Work out the finished part from the listing and answer in its coordinate system (mm). A direction names the side the tool comes from. Coordinates: 2 decimals unless noted, no trailing zeros. Order: outer loops, then holes, each group sorted by start corner. A loop starts at its lowest first (then second) coordinate and runs counter-clockwise, first axis right, second up. Notation, with made-up numbers: (5, -22) -> (9, -22) arc R21 cw to (9, -6) -> close; hole circle Ø2 at (17.25, -20). An arc over 180 degrees is marked (long way). Use one line per item in the form item = value.
from build123d import *

# Parameters (mm, degrees)
BOSS_EXTRUDE1_DEPTH  = 15
CUT_EXTRUDE2_REACH   = 8.6
SKETCH3_R            = 1.595559434
CUT_EXTRUDE5_START   = -3.6
SKETCH3_6_R          = 1.595559434
CUT_EXTRUDE5_DEPTH   = 2.6
CUT_EXTRUDE3_REACH   = 5
SKETCH4_R            = 1.5
BOSS_EXTRUDE10_DEPTH = 2.5
CUT_EXTRUDE1_DEPTH   = 10.6


with BuildPart() as part:
    # Sketch1 → Boss-Extrude1 (new body)
    with BuildSketch(Plane.ZY.offset(20.222709888)):
        with BuildLine():
            Line((144.27017666, 37.109962519), (144.27017666, 13.209962519))
            Line((144.27017666, 13.209962519), (137.68267666, 13.209962519))
            Line((137.68267666, 13.209962519), (137.68267666, 10.209962519))
            Line((137.68267666, 10.209962519), (145.433552955, 10.209962519))
            ThreePointArc((145.433552955, 10.209962519), (146.341426982, 10.902339978), (147.27017666, 11.566452794))
            Line((147.27017666, 11.566452794), (147.27017666, 43.709962519))
            Line((147.27017666, 43.709962519), (137.67017666, 43.709962519))
            Line((137.67017666, 43.709962519), (137.67017666, 37.109962519))
            Line((137.67017666, 37.109962519), (144.27017666, 37.109962519))
        make_face()
    extrude(amount=-BOSS_EXTRUDE1_DEPTH)

    # Sketch3 → Cut-Extrude2 (cut, up to next)
    with BuildSketch(Plane.XZ.offset(-37.109962519), mode=Mode.PRIVATE) as cut_extrude2_sk1:
        with Locations((-16.635209888, 140.97017666)):
            Circle(SKETCH3_R)
    cut_extrude2_tool1 = extrude(cut_extrude2_sk1.sketch, amount=-CUT_EXTRUDE2_REACH, mode=Mode.PRIVATE) & part.part
    add(cut_extrude2_tool1.solids().sort_by_distance((-16.63521, 37.109963, 140.970177))[0], mode=Mode.SUBTRACT)

    # Sketch3<6> → Cut-Extrude5 (cut)
    with BuildSketch(Plane.XZ.offset(-37.109962519).offset(CUT_EXTRUDE5_START)):
        Polygon((-19.485209888, 139.324728393), (-16.635209888, 137.679280126), (-13.785209888, 139.324728393), (-13.785209888, 142.615624927), (-16.635209888, 144.261073195), (-19.485209888, 142.615624927), align=None)
        with Locations((-16.635209888, 140.97017666)):
            Circle(SKETCH3_6_R, mode=Mode.SUBTRACT)
        Polygon((-13.785209888, 139.324728393), (-16.635209888, 137.679280126), (-19.485209888, 139.324728393), (-19.485209888, 137.67017666), (-13.785209888, 137.67017666), align=None)
        with Locations((-16.635209888, 140.97017666)):
            Circle(SKETCH3_6_R)
    extrude(amount=CUT_EXTRUDE5_DEPTH, mode=Mode.SUBTRACT)

    # Sketch4 → Cut-Extrude3 (cut, up to next)
    with BuildSketch(Plane(origin=(0, 13.209962519, 0), x_dir=(1, 0, 0), z_dir=(0, 1, 0)), mode=Mode.PRIVATE) as cut_extrude3_sk1:
        with Locations((-16.431813353, -141.42017666)):
            Circle(SKETCH4_R)
    cut_extrude3_tool1 = extrude(cut_extrude3_sk1.sketch, amount=-CUT_EXTRUDE3_REACH, mode=Mode.PRIVATE) & part.part
    add(cut_extrude3_tool1.solids().sort_by_distance((-16.431813, 13.209963, 141.420177))[0], mode=Mode.SUBTRACT)
    # Sketch4 → Cut-Extrude3 (cut, up to next)
    with BuildSketch(Plane(origin=(0, 13.209962519, 0), x_dir=(1, 0, 0), z_dir=(0, 1, 0)), mode=Mode.PRIVATE) as cut_extrude3_sk2:
        with Locations((-9.013606422, -141.42017666)):
            Circle(SKETCH4_R)
    cut_extrude3_tool2 = extrude(cut_extrude3_sk2.sketch, amount=-CUT_EXTRUDE3_REACH, mode=Mode.PRIVATE) & part.part
    add(cut_extrude3_tool2.solids().sort_by_distance((-9.013606, 13.209963, 141.420177))[0], mode=Mode.SUBTRACT)

    # Sketch11 → Boss-Extrude10 (add)
    with BuildSketch(Plane(origin=(0, 13.209962519, 0), x_dir=(1, 0, 0), z_dir=(0, 1, 0))):
        Polygon((-18.077261621, -144.27017666), (-19.722709888, -141.42017666), (-18.077261621, -138.57017666), (-14.786365086, -138.57017666), (-13.140916819, -141.42017666), (-14.786365086, -144.27017666), (-10.659054689, -144.27017666), (-12.304502957, -141.42017666), (-10.659054689, -138.57017666), (-7.368158155, -138.57017666), (-5.722709888, -141.42017666), (-7.368158155, -144.27017666), (-5.222709888, -144.27017666), (-5.222709888, -137.68267666), (-20.222709888, -137.68267666), (-20.222709888, -144.27017666), align=None)
    extrude(amount=BOSS_EXTRUDE10_DEPTH)

    # Sketch2 → Cut-Extrude1 (cut, through all)
    with BuildSketch(Plane.XY.offset(147.27017666)):
        Polygon((-12.972709888, 43.709962519), (-5.222709888, 15.709962519), (-5.222709888, 43.709962519), align=None)
    extrude(amount=-CUT_EXTRUDE1_DEPTH, mode=Mode.SUBTRACT)


solid = part.part
(1) Straight lines are drawn through the part: line 1 along X through (y, z) = (13.5, 142.5); line 2 along Y through (x, z) = (-6.75, 143.75); line 3 along Y through (x, z) = (-9, 143.25). For each, find the intervals that lie inside material, in ascending order.
Data:
line_1 = -20.22 to -19.1, -13.76 to -11.68, -6.35 to -5.22
line_2 = 10.21 to 15.71
line_3 = 10.21 to 13.21
(2) Which of the six approach directions +Z, -Z, +X, -X, +Y, -Y give full straight-line access (tool end or side, diameter ignored) to faces 1 (the flat face through (-18.912, 14.442, 140.015)), 2 (the cylindrical face through (-9.209, 11.731, 139.933)), 3 (the flat face through (-19.485, 39, 140)), 4 (the cylindrical face through (-16.843, 37.603, 142.552))?
Data:
face_1 = none
face_2 = +Y, -Y
face_3 = -Z
face_4 = +Y
(3) Each of these flat-tipped pins is pushed along its axis until it touches: P1, Ø1.3, axis at y = 39, z = 139, coming from the +X side; P2, Ø2, axis at x = -10, y = 34.5, coming from the +Z side; P3, Ø2.5, axis at x = -9.01, z = 141.42, coming from the -Y side; P4, Ø2, axis at y = 39, z = 142, coming from the +X side. Where does it stop, or does it pass through?
Data:
P1 = -11.49
P2 = 147.27
P3 = through
P4 = -11.39
(4) Section C-C on x = -9 is taken. Write down the section's boundary in (y, z), plus the area to 4 significant figures.
Data:
outline = (10.21, 137.68) -> (15.71, 137.68) -> (15.71, 138.57) -> (13.21, 138.57) -> (13.21, 139.92) -> (10.21, 139.92) -> close; (10.21, 142.92) -> (13.21, 142.92) -> (13.21, 144.27) -> (29.36, 144.27) -> (29.36, 147.27) -> (11.57, 147.27) arc R37.1 cw to (10.21, 145.43) -> close
area = 69.15 mm²
(5) Section D-D on x = -15.5 is taken. Write down the section's boundary in (y, z).
Data:
outline = (10.21, 137.68) -> (15.71, 137.68) -> (15.71, 138.57) -> (13.21, 138.57) -> (13.21, 140.24) -> (10.21, 140.24) -> close; (10.21, 142.6) -> (13.21, 142.6) -> (13.21, 144.27) -> (37.11, 144.27) -> (37.11, 142.09) -> (38.11, 142.09) -> (38.11, 143.61) -> (40.71, 143.61) -> (40.71, 142.09) -> (43.71, 142.09) -> (43.71, 147.27) -> (11.57, 147.27) arc R37.1 cw to (10.21, 145.43) -> close; (37.11, 137.67) -> (38.11, 137.67) -> (38.11, 139.85) -> (37.11, 139.85) -> close; (40.71, 137.67) -> (43.71, 137.67) -> (43.71, 139.85) -> (40.71, 139.85) -> close
(6) Section A-A on y = 14 is taken. Write down the section's boundary in (x, z).
Data:
outline = (-20.22, 137.68) -> (-5.22, 137.68) -> (-5.22, 147.27) -> (-20.22, 147.27) -> close; hole (-19.72, 141.42) -> (-18.08, 138.57) -> (-14.79, 138.57) -> (-13.14, 141.42) -> (-14.79, 144.27) -> (-18.08, 144.27) -> close; hole (-12.3, 141.42) -> (-10.66, 138.57) -> (-7.37, 138.57) -> (-5.72, 141.42) -> (-7.37, 144.27) -> (-10.66, 144.27) -> close
(7) The mould has two halves that part along X. Classify faces 5 (the flat face through (-13, 15.71, 140)), 6 (the cylindrical face through (-16.843, 42.189, 142.552)), 7 (the flat face through (-10.013, 33.017, 144.671)): released by +X, released by -X, zero draft, split by the parting line, or undercut.
Data:
face_5 = zero draft
face_6 = undercut
face_7 = released by +X
(8) Section B-B on z = 143.25 is taken. Write down the section's boundary in (x, y), plus the area to 3 significant figures.
Data:
outline = (-20.22, 10.21) -> (-5.22, 10.21) -> (-5.22, 15.71) -> (-6.78, 15.71) -> (-6.78, 13.21) -> (-11.25, 13.21) -> (-11.25, 15.71) -> (-14.2, 15.71) -> (-14.2, 13.21) -> (-18.67, 13.21) -> (-18.67, 15.71) -> (-20.22, 15.71) -> close; (-20.22, 37.11) -> (-11.15, 37.11) -> (-12.97, 43.71) -> (-20.22, 43.71) -> close; hole (-18.39, 38.11) -> (-14.88, 38.11) -> (-14.88, 40.71) -> (-18.39, 40.71) -> close
area = 105 mm²
